Could you check a few things on this drawing? It's one solid part, dimensions in mm from its lowest x, y, z. A direction names the side the tool comes from. Round coordinates to 2 decimals unless told otherwise and drop trailing zeros. Write each loop counter-clockwise with the first axis right and the second up, starting at its lowest first coordinate (ties: lowest second). Pieces come first, ordered by that corner, then holes. Notation, with made-up numbers: M 23.25,59 L 53.25,59 A8 ccw 53.25,67 Z; hole C -4.75,77 d2. An arc over 180 degrees is marked long. One line per item, written item: value. Start each with the question number.
(1) If I drill on L1, parallel to Z at x = 4.5, y = 3.75; L2, parallel to X at y = 2.75, z = 5; L3, parallel to X at y = 3.25, z = 3.25, over which ranges is the centre line in solid material (lowest first)?
(2) I want a section at B-B on y = 5.25. Please give me the cut outline in (x, z).
(3) Thinking about a two-plate mould opening in X: for the marked faces 1, 2 and 3, which applies, released by +X, released by -X, zero draft, split by the parting line, or undercut?
(4) I want a section at A-A on y = 2. Please give me the cut outline in (x, z), and give its area (3 significant figures).
(5) I'm going to push a flat-ended pin straight in: pin 1 Ø3 at (x, z) = (12, 6.5) entering from +Y. Where does the tip first touch, or does it pass through?
(6) Which directions (+Z, -Z, +X, -X, +Y, -Y) give clear straight access to the entire face, cutting with the end or side of a thin tool? Please do the marked faces 4 and 5.
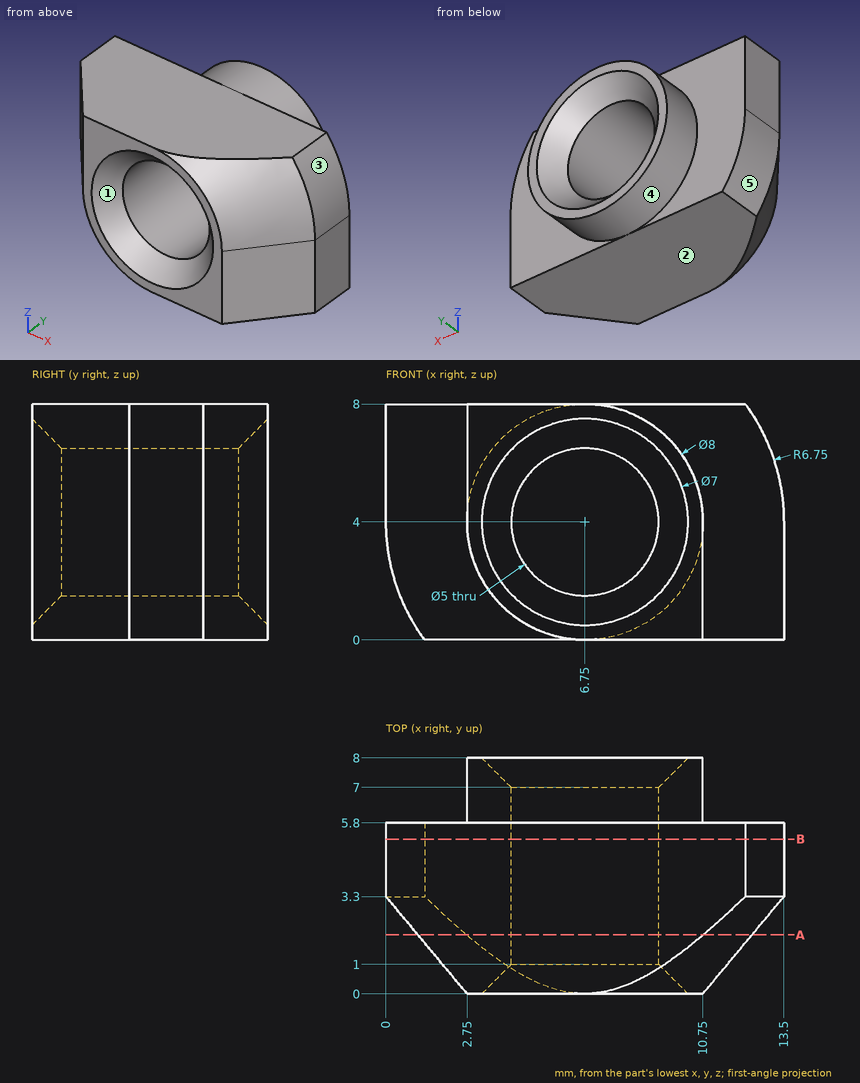
Found:
1. L1: z = 0 to 2.91, 5.09 to 8
1. L2: x = 0.46 to 4.46, 9.04 to 12.96
1. L3: x = 0.08 to 4.37, 9.13 to 13.46
2. outline: M 0,4 A6.75 ccw 1.31,0 L 13.5,0 L 13.5,4 A6.75 ccw 12.19,8 L 0,8 Z; hole C 6.75,4 d5
3. face 1: undercut
3. face 2: zero draft
3. face 3: released by +X
4. outline: M 1.08,4 A5.67 ccw 2.74,0 L 12.42,0 L 12.42,4 A5.67 ccw 10.76,8 L 1.08,8 Z; hole C 6.75,4 d5
4. area: 66.9 mm²
5. pin 1: stops at y = 5.8
6. face 4: +Y
6. face 5: -Z, -X, +Y, -Y
